Here's how the part is built. I have some questions about the finished solid (model axes, mm). A direction names the side the tool comes from. Round coordinates to 2 decimals unless told otherwise and drop trailing zeros. Write each loop counter-clockwise with the first axis right and the second up, starting at its lowest first coordinate (ties: lowest second). Pieces come first, ordered by that corner, then holes. Notation, with made-up numbers: (-11, -3) -> (37, -3) arc R16 ccw to (37, 21) -> close; hole circle Ø9 at (-26.75, 18). An arc over 180 degrees is marked (long way). Put each result on its own line as item: value. Start each with the question number.
1) I want a section at C-C, the plane y = 15.5. List the corners of the cut face in (x, z) for me, then the cut area to 3 significant figures.
2) I want a section at D-D, the plane x = -26.5. List the corners of the cut face in (y, z) for me, then the cut area to 3 significant figures.
3) Will these pins go through, and if not, where does the flat tip stop? P1, Ø5, axis at x = -42, z = -48, coming from the -Y side; P2, Ø3, axis at x = -26.5, y = 15.5, coming from the -Z side; P3, Ø3, axis at x = 6, y = -2, coming from the -Z side; P4, Ø4.5, axis at x = -28, z = -61, coming from the -Y side.
4) Which directions (+Z, -Z, +X, -X, +Y, -Y) give clear straight access to the entire face, cutting with the end or side of a thin tool? Please do faces 4 (the flat face through (-33, 3, -60)), 5 (the flat face through (-62.5, -3, -3)), 6 (the flat face through (-33, 12, -67.3)), 7 (the cylindrical face through (-26.68, 16.89, 45.53)), 8 (the flat face through (0, 10, -49)).
5) I want a section at B-B, the plane x = 53. List the corners of the cut face in (y, z) for me.
6) We'd pull the mould along Z, two halves only. Please class faces 1 (the flat face through (0, -3, 46.5)), 2 (the flat face through (-3.5, 12, -60)), 3 (the flat face through (-27, 15, -62.3)): released by +Z, released by -Z, zero draft, split by the parting line, or undercut.
7) I want a section at A-A, the plane z = -34.5. List the corners of the cut face in (x, y) for me.
8) If I drill on line 1 along Z through (x, y) = (-11, 8.25); line 2 along X through (y, z) = (18.5, 24.5); line 3 along Z through (x, y) = (45.5, 15.5), over which ranges is the centre line in solid material (lowest first)? Write a range as [from, to].
from build123d import *

# Parameters (mm, degrees)
F1_W      = 129
F1_H      = 100.5
F1_W_2    = 127
F1_H_2    = 98.5
F2_DEPTH  = 6
F3_W      = 129
F3_H      = 100.5
F3_W_2    = 121
F3_H_2    = 92.5
F4_DEPTH  = 20
F5_W      = 60
F5_H      = 14.3
F6_DEPTH  = 17
F7_R      = 1.4
F8_DEPTH  = 7.9
F9_R      = 1.4
F10_DEPTH = 5


with BuildPart() as f2:
    # F1 (on Front) → F2 (new body)
    with BuildSketch(Plane.XZ):
        with Locations((1, -2.75)):
            Rectangle(F1_W, F1_H)
        with Locations((1, -2.75)):
            Rectangle(F1_W_2, F1_H_2, mode=Mode.SUBTRACT)
    extrude(amount=F2_DEPTH)

    # F3 (on Front) → F4 (join)
    with BuildSketch(Plane.XZ):
        with Locations((1, -2.75)):
            Rectangle(F3_W, F3_H)
        with Locations((1, -2.75)):
            Rectangle(F3_W_2, F3_H_2, mode=Mode.SUBTRACT)
    extrude(amount=-F4_DEPTH)

    # F5 (on face) → F6 (join)
    with BuildSketch(Plane(origin=(0, 20, 0), x_dir=(-1, 0, 0), z_dir=(0, 1, 0))):
        with Locations((33.5, -60.15)):
            Rectangle(F5_W, F5_H)
    extrude(amount=-F6_DEPTH)

    # F7 (on face) → F8 (cut)
    with BuildSketch(Plane.XY.offset(47.5)):
        with Locations((-26.5, 15.5)):
            Circle(F7_R)
        with Locations((32.5, 15.5)):
            Circle(F7_R)
    extrude(amount=-F8_DEPTH, mode=Mode.SUBTRACT)

    # F9 (on face) → F10 (cut)
    with BuildSketch(Plane(origin=(0, 0, -67.3), x_dir=(1, 0, 0), z_dir=(0, 0, -1))):
        with Locations((-26.5, -15.5)):
            Circle(F9_R)
    extrude(amount=-F10_DEPTH, mode=Mode.SUBTRACT)


solid = f2.part
Findings:
1. outline: (-63.5, -67.3) -> (-27.9, -67.3) -> (-27.9, -62.3) -> (-25.1, -62.3) -> (-25.1, -67.3) -> (-3.5, -67.3) -> (-3.5, -53) -> (65.5, -53) -> (65.5, 47.5) -> (33.9, 47.5) -> (33.9, 43.5) -> (61.5, 43.5) -> (61.5, -49) -> (-59.5, -49) -> (-59.5, 43.5) -> (-27.9, 43.5) -> (-27.9, 47.5) -> (-63.5, 47.5) -> close; (-25.1, 43.5) -> (31.1, 43.5) -> (31.1, 47.5) -> (-25.1, 47.5) -> close
1. area: 2,590 mm2
2. outline: (-6, -53) -> (3, -53) -> (3, -67.3) -> (14.1, -67.3) -> (14.1, -62.3) -> (16.9, -62.3) -> (16.9, -67.3) -> (20, -67.3) -> (20, -49) -> (0, -49) -> (0, -52) -> (-6, -52) -> close; (-6, 46.5) -> (0, 46.5) -> (0, 43.5) -> (14.1, 43.5) -> (14.1, 47.5) -> (-6, 47.5) -> close; (16.9, 43.5) -> (20, 43.5) -> (20, 47.5) -> (16.9, 47.5) -> close
2. area: 390 mm2
3. P1: stops at y = 0
3. P2: stops at z = -67.3
3. P3: stops at z = -53
3. P4: stops at y = 3
4. face 4: -Z, +X, -X, -Y
4. face 5: -Y
4. face 6: -Z, +X, -X, +Y, -Y
4. face 7: +Z
4. face 8: +Y, -Y
5. outline: (-6, -53) -> (20, -53) -> (20, -49) -> (0, -49) -> (0, -52) -> (-6, -52) -> close; (-6, 46.5) -> (0, 46.5) -> (0, 43.5) -> (20, 43.5) -> (20, 47.5) -> (-6, 47.5) -> close
6. face 1: undercut
6. face 2: zero draft
6. face 3: released by -Z
7. outline: (-63.5, -6) -> (-62.5, -6) -> (-62.5, 0) -> (-59.5, 0) -> (-59.5, 20) -> (-63.5, 20) -> close; (61.5, 0) -> (64.5, 0) -> (64.5, -6) -> (65.5, -6) -> (65.5, 20) -> (61.5, 20) -> close
8. line 1: z = [-67.3, -49], [43.5, 47.5]
8. line 2: x = [-63.5, -59.5], [61.5, 65.5]
8. line 3: z = [-53, -49], [43.5, 47.5]
